from build123d import *

# Parameters (mm, degrees)
MAIN_DEPTH   = 6.35
ODROID_REACH = 242.916
REG_DEPTH    = 6.35
SKETCH10_W   = 6
SKETCH10_H   = 3
BAT_DEPTH    = 6.35
SKETCH11_R   = 1.75
MOUNT_DEPTH  = 6.35
CAMERA_DEPTH = 6.35


with BuildPart() as part:
    # Sketch1 → main (new body)
    with BuildSketch(Plane(origin=(0, 0, 0), x_dir=(1, 0, 0), z_dir=(0, 1, 0))):
        with BuildLine():
            Line((-10, 0), (-150, 0))
            ThreePointArc((-150, 0), (-157.071067812, 2.928932188), (-160, 10))
            Line((-160, 10), (-160, 170))
            ThreePointArc((-160, 170), (-157.071067812, 177.071067812), (-150, 180))
            Line((-150, 180), (-10, 180))
            ThreePointArc((-10, 180), (-2.928932188, 177.071067812), (0, 170))
            Line((0, 170), (0, 10))
            ThreePointArc((0, 10), (-2.928932188, 2.928932188), (-10, 0))
        make_face()
    extrude(amount=MAIN_DEPTH)

    # Sketch8 → odroid (cut, up to next)
    with BuildSketch(Plane.XZ, mode=Mode.PRIVATE) as odroid_sk1:
        with BuildLine():
            Line((-96.25, -147.5), (-96.25, -152.5))
            ThreePointArc((-96.25, -152.5), (-98, -154.25), (-99.75, -152.5))
            Line((-99.75, -152.5), (-99.75, -147.5))
            ThreePointArc((-99.75, -147.5), (-98, -145.75), (-96.25, -147.5))
        make_face()
    odroid_tool1 = extrude(odroid_sk1.sketch, amount=-ODROID_REACH, mode=Mode.PRIVATE) & part.part
    # Sketch8 → odroid (cut, up to next)
    with BuildSketch(Plane.XZ, mode=Mode.PRIVATE) as odroid_sk2:
        with BuildLine():
            Line((-96.25, -71.5), (-96.25, -76.5))
            ThreePointArc((-96.25, -76.5), (-98, -78.25), (-99.75, -76.5))
            Line((-99.75, -76.5), (-99.75, -71.5))
            ThreePointArc((-99.75, -71.5), (-98, -69.75), (-96.25, -71.5))
        make_face()
    odroid_tool2 = extrude(odroid_sk2.sketch, amount=-ODROID_REACH, mode=Mode.PRIVATE) & part.part
    # Sketch8 → odroid (cut, up to next)
    with BuildSketch(Plane.XZ, mode=Mode.PRIVATE) as odroid_sk3:
        with BuildLine():
            Line((-148.25, -147.5), (-148.25, -152.5))
            ThreePointArc((-148.25, -152.5), (-150, -154.25), (-151.75, -152.5))
            Line((-151.75, -152.5), (-151.75, -147.5))
            ThreePointArc((-151.75, -147.5), (-150, -145.75), (-148.25, -147.5))
        make_face()
    odroid_tool3 = extrude(odroid_sk3.sketch, amount=-ODROID_REACH, mode=Mode.PRIVATE) & part.part
    # Sketch8 → odroid (cut, up to next)
    with BuildSketch(Plane.XZ, mode=Mode.PRIVATE) as odroid_sk4:
        with BuildLine():
            Line((-148.25, -71.5), (-148.25, -76.5))
            ThreePointArc((-148.25, -76.5), (-150, -78.25), (-151.75, -76.5))
            Line((-151.75, -76.5), (-151.75, -71.5))
            ThreePointArc((-151.75, -71.5), (-150, -69.75), (-148.25, -71.5))
        make_face()
    odroid_tool4 = extrude(odroid_sk4.sketch, amount=-ODROID_REACH, mode=Mode.PRIVATE) & part.part
    add(odroid_tool1.solids().sort_by_distance((-98, 0, -150))[0], mode=Mode.SUBTRACT)
    add(odroid_tool2.solids().sort_by_distance((-98, 0, -74))[0], mode=Mode.SUBTRACT)
    add(odroid_tool3.solids().sort_by_distance((-150, 0, -150))[0], mode=Mode.SUBTRACT)
    add(odroid_tool4.solids().sort_by_distance((-150, 0, -74))[0], mode=Mode.SUBTRACT)

    # Sketch9 → reg (cut)
    with BuildSketch(Plane.XZ):
        with BuildLine():
            Line((-58, -104.6), (-64, -104.6))
            ThreePointArc((-64, -104.6), (-65.6, -103), (-64, -101.4))
            Line((-64, -101.4), (-58, -101.4))
            ThreePointArc((-58, -101.4), (-56.4, -103), (-58, -104.6))
        make_face()
        with BuildLine():
            Line((-16, -104.6), (-22, -104.6))
            ThreePointArc((-22, -104.6), (-23.6, -103), (-22, -101.4))
            Line((-22, -101.4), (-16, -101.4))
            ThreePointArc((-16, -101.4), (-14.4, -103), (-16, -104.6))
        make_face()
    extrude(amount=-REG_DEPTH, mode=Mode.SUBTRACT)

    # Sketch10 → bat (cut)
    with BuildSketch(Plane.XZ):
        with Locations((-52, -58.5)):
            Rectangle(SKETCH10_W, SKETCH10_H)
        with Locations((-108, -13.5)):
            Rectangle(SKETCH10_W, SKETCH10_H)
        with Locations((-108, -58.5)):
            Rectangle(SKETCH10_W, SKETCH10_H)
        with Locations((-52, -13.5)):
            Rectangle(SKETCH10_W, SKETCH10_H)
    extrude(amount=-BAT_DEPTH, mode=Mode.SUBTRACT)

    # Sketch11 → mount (cut)
    with BuildSketch(Plane.XZ):
        with Locations(Location((-67.5, -167.5, 0), (0, 0, 270))):
            Circle(SKETCH11_R)
        with Locations(Location((-42.5, -167.5, 0), (0, 0, 270))):
            Circle(SKETCH11_R)
        with Locations(Location((-117.5, -12.5, 0), (0, 0, 270))):
            Circle(SKETCH11_R)
        with Locations(Location((-92.5, -167.5, 0), (0, 0, 90))):
            Circle(SKETCH11_R)
        with Locations(Location((-92.5, -12.5, 0), (0, 0, 270))):
            Circle(SKETCH11_R)
        with Locations(Location((-42.5, -12.5, 0), (0, 0, 90))):
            Circle(SKETCH11_R)
        with Locations(Location((-67.5, -12.5, 0), (0, 0, 90))):
            Circle(SKETCH11_R)
        with Locations(Location((-117.5, -167.5, 0), (0, 0, 90))):
            Circle(SKETCH11_R)
    extrude(amount=-MOUNT_DEPTH, mode=Mode.SUBTRACT)

    # Sketch12 → camera (cut)
    with BuildSketch(Plane.XZ):
        with BuildLine():
            Line((-48.5, -173.5), (-56.5, -173.5))
            ThreePointArc((-56.5, -173.5), (-58, -172), (-56.5, -170.5))
            Line((-56.5, -170.5), (-48.5, -170.5))
            ThreePointArc((-48.5, -170.5), (-47, -172), (-48.5, -173.5))
        make_face()
        with BuildLine():
            Line((-111.5, -173.5), (-103.5, -173.5))
            ThreePointArc((-103.5, -173.5), (-102, -172), (-103.5, -170.5))
            Line((-103.5, -170.5), (-111.5, -170.5))
            ThreePointArc((-111.5, -170.5), (-113, -172), (-111.5, -173.5))
        make_face()
    extrude(amount=-CAMERA_DEPTH, mode=Mode.SUBTRACT)


solid = part.part
Geometry: final body of the model. Coordinates: model frame, mm. A direction names the side the tool comes from. Give positions to 0.01 mm unless a question says otherwise; leave off trailing zeros. Write each loop counter-clockwise with the first axis right and the second up, starting at its lowest first coordinate (ties: lowest second). Pieces come first, ordered by that corner, then holes.
(1) Access query for faces 4 (the flat face through (-52, 3, -12)), 5 (the flat face through (-79, 0, -91)). Directions: +Z, -Z, +X, -X, +Y, -Y. A direction counts if a zero-diameter tool reaches every point of the face in a straight line with its end or side. Return the directions, or none.
(2) Mould query, pull axis X, two halves, no side actions, for faces 1 (the flat face through (-61, 3, -104.6)), 2 (the cylindrical face through (-157.15, 3.13, -176.99)), 3 (the flat face through (-79, 6.35, -91)). Classes: released by +X, released by -X, zero draft, split by the parting line, or undercut.
(3) Cut plane A-A, the plane x = -60. Return loops of the section in (y, z).
(4) First-contact query: P1, Ø5, axis at x = -112, z = -106, coming from the -Y side. Flat tip, straight axial feed; report the tip coordinate or a pass-through.
(5) Ray query, line 1 (Z direction, x = -92.5, y = 5); line 2 (Z direction, x = -94, y = 5.5); line 3 (Z direction, x = -109, y = 1). Return the intervals inside material, ascending.
(6) Cut plane B-B, the plane y = 1.5. Give the number of separate pieces and of enclosed holes in the cut face, then the cut area to 3 significant figures.
Values follow:
1. face 4: +Y, -Y
1. face 5: +Z, -Z, +X, -X, -Y
2. face 1: undercut
2. face 2: released by -X
2. face 3: zero draft
3. outline: (0, -180) - (6.35, -180) - (6.35, -104.6) - (0, -104.6) - close; (0, -101.4) - (6.35, -101.4) - (6.35, 0) - (0, 0) - close
4. P1: stops at y = 0
5. line 1: z = -180 to -169.25, -165.75 to -14.25, -10.75 to 0
5. line 2: z = -180 to -168.4, -166.6 to -13.4, -11.6 to 0
5. line 3: z = -180 to -173.5, -170.5 to -60, -57 to -15, -12 to 0
6. separate pieces: 1
6. enclosed holes: 20
6. area: 28,300 mm2
